Verification items for the finished model (mm, model axes). A direction names the side the tool comes from. Give positions to 0.01 mm unless a question says otherwise; leave off trailing zeros. Loops run counter-clockwise (first coordinate to the right, second up) from the corner with the lowest first, then second, coordinate; pieces in that order, holes last. Notation, with made-up numbers: M 56,82.25 L 75,82.25 A18 ccw 75,102.25 Z; hole C 58.5,-3.75 d3. An arc over 180 degrees is marked long. Answer in a Markdown table with one row per item.
```python
from build123d import *

# Parameters (mm, degrees)
F0_W          = 70
F0_H          = 60
F1_DEPTH      = 5
F2_R          = 4
F3_DEPTH      = 3
F4_R          = 1.5
F5_DEPTH      = 3.001
F5_DEPTH_BACK = 5
F6_DEPTH      = 9.85
F7_DEPTH      = 9.85
F8_DEPTH      = 5.11
F9_DEPTH      = 5.11
F10_R         = 2
F11_DEPTH     = 5
F12_R         = 4
F13_DEPTH     = 3
F15_DEPTH     = 2.5


with BuildPart() as f1:
    # F0 (on Top) → F1 (new body)
    with BuildSketch(Plane.XY):
        Rectangle(F0_W, F0_H)
    extrude(amount=F1_DEPTH)

    # F2 (on face) → F3 (join)
    with BuildSketch(Plane.XY.offset(5)):
        with Locations((-23.7, 23.1)):
            Circle(F2_R)
        with Locations((-25, -25.1)):
            Circle(F2_R)
        with Locations((27.1, 7.9)):
            Circle(F2_R)
        with Locations((27.1, -20)):
            Circle(F2_R)
    extrude(amount=F3_DEPTH)

    # F4 (on face) → F5 (cut, two sides)
    with BuildSketch(Plane.XY.offset(5)) as f5_sk:
        with Locations((-23.7, 23.1)):
            Circle(F4_R)
        with Locations((27.1, 7.9)):
            Circle(F4_R)
        with Locations((27.1, -20)):
            Circle(F4_R)
        with Locations((-25, -25.1)):
            Circle(F4_R)
    extrude(amount=F5_DEPTH, mode=Mode.SUBTRACT)
    extrude(f5_sk.sketch, amount=-F5_DEPTH_BACK, mode=Mode.SUBTRACT)

    # F6 (add): a face of the model
    f6_faces = [f1.faces().sort_by_distance(p)[0] for p in [
        (0, -30, 2.5),
    ]]
    extrude(f6_faces, amount=F6_DEPTH)

    # F7 (add): a face of the model
    f7_faces = [f1.faces().sort_by_distance(p)[0] for p in [
        (0, 30, 2.5),
    ]]
    extrude(f7_faces, amount=F7_DEPTH)

    # F8 (add): a face of the model
    f8_faces = [f1.faces().sort_by_distance(p)[0] for p in [
        (35, 0, 2.5),
    ]]
    extrude(f8_faces, amount=F8_DEPTH)

    # F9 (add): a face of the model
    f9_faces = [f1.faces().sort_by_distance(p)[0] for p in [
        (-35, 0, 2.5),
    ]]
    extrude(f9_faces, amount=F9_DEPTH)

    # F10 (on face) → F11 (cut)
    with BuildSketch(Plane.XY.offset(5)):
        with Locations((-12.11, 0.15)):
            Circle(F10_R)
        with Locations((-12.11, 24.15)):
            Circle(F10_R)
        with Locations((17.89, 24.15)):
            Circle(F10_R)
        with Locations((17.89, 0.15)):
            Circle(F10_R)
    extrude(amount=-F11_DEPTH, mode=Mode.SUBTRACT)

    # F12 (on face) → F13 (cut)
    with BuildSketch(Plane.XY.offset(5)):
        with Locations((-12.11, 0.15)):
            Circle(F12_R)
        with Locations((-12.11, 24.15)):
            Circle(F12_R)
        with Locations((17.89, 24.15)):
            Circle(F12_R)
        with Locations((17.89, 0.15)):
            Circle(F12_R)
    extrude(amount=-F13_DEPTH, mode=Mode.SUBTRACT)

    # F14 (on face) → F15 (cut)
    with BuildSketch(Plane(origin=(0, 0, 0), x_dir=(1, 0, 0), z_dir=(0, 0, -1))):
        Polygon((-24.6492034201, 28.2559903506), (-27.5577695278, 26.981793925), (-27.9085661076, 23.8258035744), (-25.3507965799, 21.9440096494), (-22.4422304722, 23.218206075), (-22.0914338924, 26.3741964256), align=None)
        Polygon((27.1832127793, 23.1743359883), (24.3925507836, 21.659232375), (24.3093380043, 18.4848963867), (27.0167872207, 16.8256640117), (29.8074492164, 18.340767625), (29.8906619957, 21.5151036133), align=None)
        Polygon((27.1178128759, -4.7246234814), (24.3589497063, -6.2968853377), (24.3411368304, -9.4722618563), (27.0821871241, -11.0753765186), (29.8410502937, -9.5031146623), (29.8588631696, -6.3277381437), align=None)
        Polygon((-23.1561984645, -19.9714838624), (-26.1374736836, -21.0647959868), (-26.6812752191, -24.1933121244), (-24.2438015355, -26.2285161376), (-21.2625263164, -25.1352040132), (-20.7187247809, -22.0066878756), align=None)
    extrude(amount=-F15_DEPTH, mode=Mode.SUBTRACT)


solid = f1.part
```
Item 1: Sectioned sample at D-D (y = 23.1). State how many separate pieces and enclosed holes the cut face has, and give its area (3 significant figures).
Reported:
| item | result |
|---|---|
| separate pieces | 4 |
| enclosed holes | 0 |
| area | 335 mm^2 |
Item 2: Go/stop test with flat-tipped pins: pin 1 (5 mm diameter, centred on x = -12.11, y = 0.15, fed in from +Z); pin 2 (1.7 mm diameter, centred on x = -24, y = -25.5, fed in from -Z); pin 3 (9 mm diameter, centred on x = 17.89, y = 24.15, fed in from +Z); pin 4 (2.5 mm diameter, centred on x = 27.1, y = -20, fed in from +Z). Record where each tip stops, or that it passes through.
Reported:
| item | result |
|---|---|
| pin 1 | stops at z = 2 |
| pin 2 | stops at z = 2.5 |
| pin 3 | stops at z = 5 |
| pin 4 | passes through |
Item 3: Sectioned sample at A-A (z = 6.75). Record the cut outline in (x, y).
Reported:
| item | result |
|---|---|
| outline | C -25,-25.1 d8; C -23.7,23.1 d8; C 27.1,-20 d8; C 27.1,7.9 d8; hole C -25,-25.1 d3; hole C -23.7,23.1 d3; hole C 27.1,-20 d3; hole C 27.1,7.9 d3 |
Item 4: Sectioned sample at B-B (y = 0.15). Record the cut outline in (x, z).
Reported:
| item | result |
|---|---|
| outline | M -40.11,0 L -14.11,0 L -14.11,2 L -16.11,2 L -16.11,5 L -40.11,5 Z; M -10.11,0 L 15.89,0 L 15.89,2 L 13.89,2 L 13.89,5 L -8.11,5 L -8.11,2 L -10.11,2 Z; M 19.89,0 L 40.11,0 L 40.11,5 L 21.89,5 L 21.89,2 L 19.89,2 Z |
Item 5: Tool access check on faces 1 (the flat face through (25.64, -17.67, 1.23)), 2 (the cylindrical face through (30.915, 9.101, 6.479)), 3 (the cylindrical face through (25.6, 7.97, 5.29)). Record the directions out of +Z, -Z, +X, -X, +Y, -Y that give a thin tool (end or side, any length) a straight path to the whole face; none if there is none.
Reported:
| item | result |
|---|---|
| face 1 | -Z |
| face 2 | +Z |
| face 3 | +Z, -Z |
Item 6: Scan lines: L1, parallel to Y at x = 27.1, z = 5.15; L2, parallel to Y at x = -12.11, z = 4.4; L3, parallel to Y at x = 27.1, z = 4. Record each from-to range of solid material in increasing order. Write a range as [from, to].
Reported:
| item | result |
|---|---|
| L1 | y = [-24, -21.5], [-18.5, -16], [3.9, 6.4], [9.4, 11.9] |
| L2 | y = [-39.85, -3.85], [4.15, 20.15], [28.15, 39.85] |
| L3 | y = [-39.85, -21.5], [-18.5, 6.4], [9.4, 39.85] |
Item 7: Sectioned sample at C-C (y = -20). Record the cut outline in (x, z).
Reported:
| item | result |
|---|---|
| outline | M -40.11,0 L 24.35,0 L 24.35,2.5 L 25.6,2.5 L 25.6,8 L 23.1,8 L 23.1,5 L -40.11,5 Z; M 28.6,2.5 L 29.85,2.5 L 29.85,0 L 40.11,0 L 40.11,5 L 31.1,5 L 31.1,8 L 28.6,8 Z |
Item 8: Release check for a two-part mould opening along Y. For faces 4 (the flat face through (-24, 21, 8)), 5 (the cylindrical face through (-13.697, -1.067, 1.014)), 6 (the cylindrical face through (-21.854, 19.551, 6.479)), 7 (the flat face through (1, 39.85, 2)) record: released by +Y, released by -Y, zero draft, split by the parting line, or undercut.
Reported:
| item | result |
|---|---|
| face 4 | zero draft |
| face 5 | undercut |
| face 6 | undercut |
| face 7 | released by +Y |
